Input: part model. Units: mm. Frame: model coordinates. A direction names the side the tool comes from. Coordinates: 2 decimals unless noted, no trailing zeros. Order: outer loops, then holes, each group sorted by start corner. A loop starts at its lowest first (then second) coordinate and runs counter-clockwise, first axis right, second up. Notation, with made-up numbers: (86.5, 45) - (96.5, 45) arc R31 ccw to (96.5, 84) - close; hole circle Ø4 at (0, -26.75). An arc over 180 degrees is marked (long way). One line per question, with ' | ' between items.
from build123d import *

# Parameters (mm, degrees)
SKETCH1_R               = 6.65
BOSS_EXTRUDE1_DEPTH     = 8.25
BOSS_EXTRUDE1_TAPER     = 20
SKETCH2_R               = 6.65
SKETCH2_R_2             = 5.45
BOSS_EXTRUDE2_DEPTH     = 1
SKETCH3_R               = 2.1
CUT_EXTRUDE1_DEPTH      = 13.51029576
CUT_EXTRUDE2_DEPTH      = 13.51029576
CUT_EXTRUDE2_DEPTH_BACK = 13.51029576
SKETCH4_W               = 15
SKETCH4_H               = 5
SKETCH5_R               = 2.1
BOSS_EXTRUDE3_DEPTH     = 8.25
CUT_EXTRUDE3_REACH      = 20.994
CUT_EXTRUDE3_START      = -1.2
CUT_EXTRUDE4_REACH      = 19.794
SKETCH7_R               = 1.15
FILLET1_SIZE            = 2


with BuildPart() as part:
    # Sketch1 → Boss-Extrude1 (new body)
    with BuildSketch(Plane.XY):
        Circle(SKETCH1_R)
    extrude(amount=BOSS_EXTRUDE1_DEPTH, taper=BOSS_EXTRUDE1_TAPER)

    # Sketch2 → Boss-Extrude2 (add)
    with BuildSketch(Plane(origin=(0, 0, 0), x_dir=(-1, 0, 0), z_dir=(0, 0, -1))):
        Circle(SKETCH2_R)
        Circle(SKETCH2_R_2, mode=Mode.SUBTRACT)
    extrude(amount=BOSS_EXTRUDE2_DEPTH)

    # Sketch3 → Cut-Extrude1 (cut, through all)
    with BuildSketch(Plane(origin=(0, 0, 0), x_dir=(-1, 0, 0), z_dir=(0, 0, -1))):
        Circle(SKETCH3_R)
    extrude(amount=-CUT_EXTRUDE1_DEPTH, mode=Mode.SUBTRACT)

    # Sketch4 → Cut-Extrude2 (cut, two sides: drawn at the far end of the back side and taken through both)
    with BuildSketch(Plane.XY.offset(-CUT_EXTRUDE2_DEPTH_BACK)):
        with Locations((0, -8.795)):
            Rectangle(SKETCH4_W, SKETCH4_H)
    extrude(amount=CUT_EXTRUDE2_DEPTH + CUT_EXTRUDE2_DEPTH_BACK, mode=Mode.SUBTRACT)

    # Sketch5 → Boss-Extrude3 (add)
    with BuildSketch(Plane.XY):
        with BuildLine():
            Line((3.647245567, 0), (3.647245567, -3.295))
            Line((3.647245567, -3.295), (9, -3.295))
            Line((9, -3.295), (9, -6.295))
            Line((9, -6.295), (-9, -6.295))
            Line((-9, -6.295), (-9, -3.295))
            Line((-9, -3.295), (-3.647245567, -3.295))
            Line((-3.647245567, -3.295), (-3.647245567, 0))
            ThreePointArc((-3.647245567, 0), (0, 3.647245567), (3.647245567, 0))
        make_face()
        with Locations(Location((0, 0, 0), (0, 0, 180))):
            Circle(SKETCH5_R, mode=Mode.SUBTRACT)
    extrude(amount=BOSS_EXTRUDE3_DEPTH)

    # Sketch6 → Cut-Extrude3 (cut, up to next)
    with BuildSketch(Plane.XZ.offset(6.295).offset(CUT_EXTRUDE3_START), mode=Mode.PRIVATE) as cut_extrude3_sk1:
        Polygon((-6.650898686, 6.457886687), (-9.095788478, 6.026786651), (-9.944889792, 3.693899965), (-8.349101314, 1.792113313), (-5.904211522, 2.223213349), (-5.055110208, 4.556100035), align=None)
    cut_extrude3_tool1 = extrude(cut_extrude3_sk1.sketch, amount=-CUT_EXTRUDE3_REACH, mode=Mode.PRIVATE) & part.part
    # Sketch6 → Cut-Extrude3 (cut, up to next)
    with BuildSketch(Plane.XZ.offset(6.295).offset(CUT_EXTRUDE3_START), mode=Mode.PRIVATE) as cut_extrude3_sk2:
        Polygon((6.650898686, 6.457886687), (5.055110208, 4.556100035), (5.904211522, 2.223213349), (8.349101314, 1.792113313), (9.944889792, 3.693899965), (9.095788478, 6.026786651), align=None)
    cut_extrude3_tool2 = extrude(cut_extrude3_sk2.sketch, amount=-CUT_EXTRUDE3_REACH, mode=Mode.PRIVATE) & part.part
    add(cut_extrude3_tool1.solids().sort_by_distance((-7.5, -5.095, 4.125))[0], mode=Mode.SUBTRACT)
    add(cut_extrude3_tool2.solids().sort_by_distance((7.5, -5.095, 4.125))[0], mode=Mode.SUBTRACT)

    # Sketch7 → Cut-Extrude4 (cut, up to next)
    with BuildSketch(Plane.XZ.offset(6.295), mode=Mode.PRIVATE) as cut_extrude4_sk1:
        with Locations((7.5, 4.125)):
            Circle(SKETCH7_R)
    cut_extrude4_tool1 = extrude(cut_extrude4_sk1.sketch, amount=-CUT_EXTRUDE4_REACH, mode=Mode.PRIVATE) & part.part
    # Sketch7 → Cut-Extrude4 (cut, up to next)
    with BuildSketch(Plane.XZ.offset(6.295), mode=Mode.PRIVATE) as cut_extrude4_sk2:
        with Locations((-7.5, 4.125)):
            Circle(SKETCH7_R)
    cut_extrude4_tool2 = extrude(cut_extrude4_sk2.sketch, amount=-CUT_EXTRUDE4_REACH, mode=Mode.PRIVATE) & part.part
    add(cut_extrude4_tool1.solids().sort_by_distance((7.5, -6.295, 4.125))[0], mode=Mode.SUBTRACT)
    add(cut_extrude4_tool2.solids().sort_by_distance((-7.5, -6.295, 4.125))[0], mode=Mode.SUBTRACT)

    # Fillet1
    # a fillet whose section is not a circle: 2 mm, written as the material it takes off along each edge
    with BuildSketch(Plane(origin=(9, 1.705, 0), x_dir=(0, 0, 1), z_dir=(0, -1, 0)), Plane(origin=(9, 1.705, 8.25), x_dir=(-1, 0, 0), z_dir=(0, -1, 0)), Plane(origin=(-9, -11.295, 0), x_dir=(0, 0, 1), z_dir=(0, 1, 0)), Plane(origin=(-9, -11.295, 8.25), x_dir=(1, 0, 0), z_dir=(0, 1, 0))) as fillet1_piece_1:
        with BuildLine():
            add(Edge.make_bspline([(FILLET1_SIZE, 0), (FILLET1_SIZE * 0.831801948466, 0), (FILLET1_SIZE * 0.663603896932, 0), (FILLET1_SIZE * 0.292893218813, FILLET1_SIZE * 0.0716919198361), (FILLET1_SIZE * 0.0716919198361, FILLET1_SIZE * 0.292893218813), (0, FILLET1_SIZE * 0.663603896932), (0, FILLET1_SIZE * 0.831801948466), (0, FILLET1_SIZE)], knots=[0, 0, 0, 0, 0, 0, 0.5, 0.5, 1, 1, 1, 1, 1, 1], degree=5))
            Line((0, FILLET1_SIZE), (0, 0))
            Line((0, 0), (FILLET1_SIZE, 0))
        make_face()
    extrude(amount=13, mode=Mode.SUBTRACT)


solid = part.part
Item 1: Section A-A on z = 3.25. Return the cut outline in (x, y) (1 decimal).
Data:
outline: (-9, -6.3) - (-8.2, -6.3) - (-8.2, -5.1) - (-9, -5.1) - close; (-6.8, -6.3) - (6.8, -6.3) - (6.8, -5.1) - (5.5, -5.1) - (5.5, -3.3) - (4.4, -3.3) arc R5.5 ccw (long way) to (-4.4, -3.3) - (-5.5, -3.3) - (-5.5, -5.1) - (-6.8, -5.1) - close; (8.2, -6.3) - (9, -6.3) - (9, -5.1) - (8.2, -5.1) - close; hole circle Ø4.2 at (0, 0)
Item 2: Draft query along Z for faces 1 (the face through (-6, -5, 0)), 2 (the face through (5, -3.295, 5)), 3 (the face through (-5.84, -4.21, 5.49)). Return one class per face: released by +Z, released by -Z, zero draft, split by the parting line, or undercut.
Data:
face 1: released by -Z | face 2: zero draft | face 3: undercut
Item 3: Section C-C on z = 5.5. Return the cut outline in (x, y) (1 decimal).
Data:
outline: (-9, -6.3) - (9, -6.3) - (9, -5.1) - (5.8, -5.1) - (5.8, -3.3) - (3.6, -3.3) - (3.6, -2.9) arc R4.6 ccw (long way) to (-3.6, -2.9) - (-3.6, -3.3) - (-5.8, -3.3) - (-5.8, -5.1) - (-9, -5.1) - close; hole circle Ø4.2 at (0, 0)
Item 4: Section B-B on x = 0. Return the cut outline in (y, z) (3 decimals), and give its area (3 significant figures).
Data:
outline: (-6.295, -1) - (-5.45, -1) - (-5.45, 0) - (-2.1, 0) - (-2.1, 8.25) - (-6.295, 8.25) - close; (2.1, 0) - (5.45, 0) - (5.45, -1) - (6.65, -1) - (6.65, 0) - (3.647, 8.25) - (2.1, 8.25) - close | area: 61.8 mm^2
Item 5: Access query for faces 4 (the face through (-5.198, 1.637, -0.493)), 5 (the face through (-7.809, -4.208, 6.254)), 6 (the face through (-3.647, -2.4, 7.3)). Directions: +Z, -Z, +X, -X, +Y, -Y. A direction counts if a zero-diameter tool reaches every point of the face in a straight line with its end or side. Return the directions, or none.
Data:
face 4: -Z | face 5: +Y | face 6: +Z, -X
Item 6: Ray query, line 1 (Y direction, x = 0, z = -0.65) (3 decimals); line 2 (X direction, y = 0, z = -0.2); line 3 (Y direction, x = -7, z = 5.75) (3 decimals). Return the intervals inside material, ascending.
Data:
line 1: -6.295 to -5.45, 5.45 to 6.65 | line 2: -6.65 to -5.45, 5.45 to 6.65 | line 3: -6.295 to -5.095
Item 7: Contact query for flat-ended pins moving along their axis: P1, Ø0.9, axis at x = 5.5, y = -5, coming from the -Z side; P2, Ø2.5, axis at y = -1.5, z = 7, coming from the -X side; P3, Ø1.5, axis at x = -3.5, z = 3.5, coming from the +Y side. Output: stop coordinate, or through.
Data:
P1: z = 0 | P2: x = -4.41 | P3: y = 4.72
